Check sheet for the drawn part. Datum: minimum x, y, z corner. Units: mm. A direction names the side the tool comes from. Coordinates: 2 decimals unless noted, no trailing zeros. Order: outer loops, then holes, each group sorted by start corner. A loop starts at its lowest first (then second) coordinate and runs counter-clockwise, first axis right, second up. Notation, with made-up numbers: (-35, -4.5) - (-31, -4.5) arc R15 ccw to (-31, -0.5) - close; hole circle Ø4 at (77, 11). An arc over 180 degrees is marked (long way). Answer as CSV lines item,"result". Start each with the question number.
1. Section check C-C (z = 35.5). Record the cut outline in (x, y), and give its area (3 significant figures).
2. Material ranges on L1, parallel to Y at x = 8, z = 42; L2, parallel to Z at x = 33, y = 31, recorded low to high. Write a range as [from, to].
3. Section check B-B (x = 48). Record the cut outline in (y, z).
4. Set-up check for the marked faces 1, 2, 3, 4 and 5: record each of +Z, -Z, +X, -X, +Y, -Y from which the full face is reachable in a straight line by a thin tool's end or side.
5. Section check A-A (y = 13). Record the cut outline in (x, z), and give its area (3 significant figures).
6. Section check D-D (x = 63.5). Record the cut outline in (y, z).
7. Go/stop test with flat-tipped pins: pin 1 (20.5 mm diameter, centred on y = 18, z = 8, fed in from -X); pin 2 (1 mm diameter, centred on x = 11.5, y = 9, fed in from -Z); pin 3 (12.5 mm diameter, centred on x = 10, z = 38, fed in from +Y); pin 4 (4 mm diameter, centred on y = 33.5, z = 23, fed in from -X). Record where each tip stops, or that it passes through.
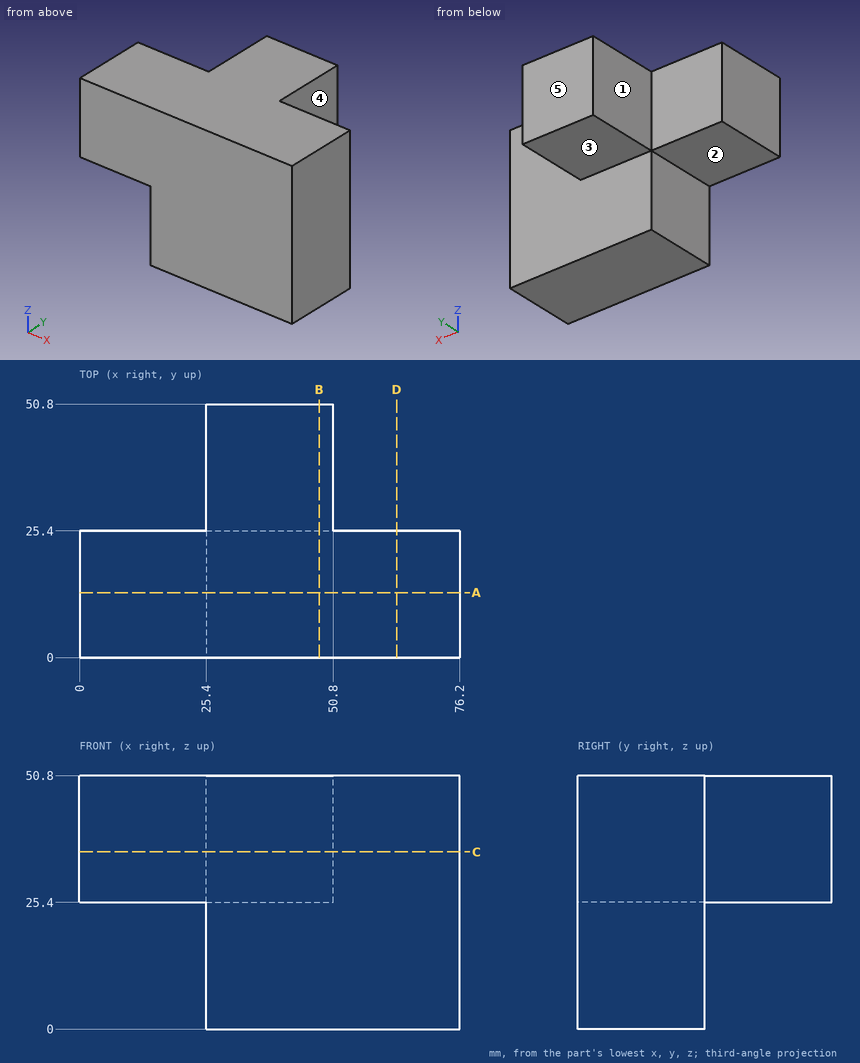
Evaluation:
1,outline,"(0, 0) - (76.2, 0) - (76.2, 25.4) - (50.8, 25.4) - (50.8, 50.8) - (25.4, 50.8) - (25.4, 25.4) - (0, 25.4) - close"
1,area,"2,580 mm²"
2,L1,"y = [0, 25.4]"
2,L2,"z = [25.4, 50.8]"
3,outline,"(0, 0) - (25.4, 0) - (25.4, 25.4) - (50.8, 25.4) - (50.8, 50.8) - (0, 50.8) - close"
4,face 1,"+Z, -Z, -X, +Y"
4,face 2,"-Z, -X, +Y, -Y"
4,face 3,"-Z, +X, -X, +Y"
4,face 4,"+Z, -Z, +X, +Y"
4,face 5,"+Z, -Z, +X, -X, +Y"
5,outline,"(0, 25.4) - (25.4, 25.4) - (25.4, 0) - (76.2, 0) - (76.2, 50.8) - (0, 50.8) - close"
5,area,"3,230 mm²"
6,outline,"(0, 0) - (25.4, 0) - (25.4, 50.8) - (0, 50.8) - close"
7,pin 1,"stops at x = 25.4"
7,pin 2,"stops at z = 25.4"
7,pin 3,"stops at y = 25.4"
7,pin 4,"passes through"
